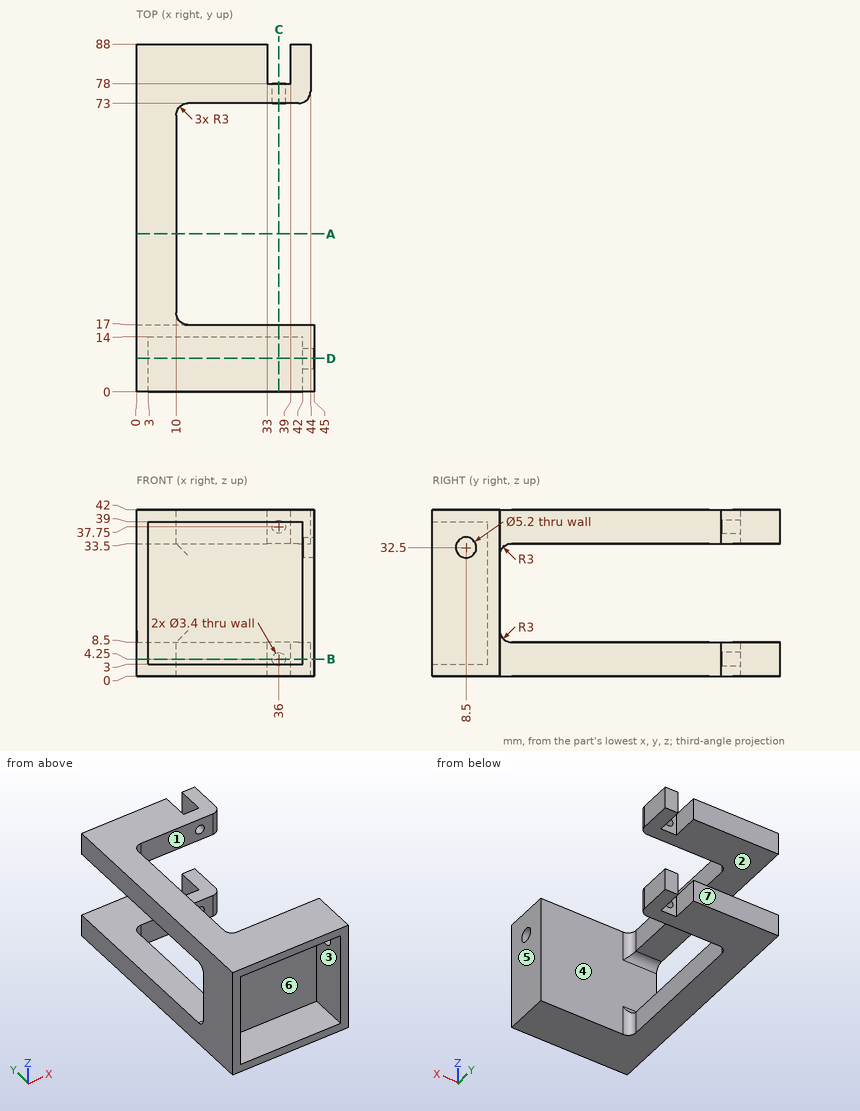
The figure shows three views and two pictorial views of one solid part (mm, origin at its lowest corner). Answer the questions. A direction names the side the tool comes from. Give positions to 0.01 mm unless a question says otherwise; leave off trailing zeros. Loops run counter-clockwise (first coordinate to the right, second up) from the corner with the lowest first, then second, coordinate; pieces in that order, holes last. Notation, with made-up numbers: (56.5, 30.25) -> (91.5, 30.25) arc R13 ccw to (91.5, 35.25) -> close; hole circle Ø7 at (43, 52). An arc over 180 degrees is marked (long way). Use a Markdown table: item, result. Add a question column.
1. Section B-B on z = 4.25 is taken. Determine the outline of the cut face in (x, y), and give its area (3 significant figures).
2. Section C-C on x = 36 is taken. Determine the outline of the cut face in (y, z).
3. Find the intervals of material crossed by probe 1 along Y at (x, z) = (32.5, 7.5); probe 2 along Y at (x, z) = (43.7, 32.5); probe 3 along Z at (x, y) = (3, 25.5), in increasing order.
4. Section D-D on y = 8.5 is taken. Determine the outline of the cut face in (x, z).
5. Determine the mould class of the marked faces 5, 6 and 7 for opening direction X: released by +X, released by -X, zero draft, split by the parting line, or undercut.
6. Flat-ended cylindrical pins translate along their axes: pin 1 Ø6 at (y, z) = (42.5, 34.5) entering from +X; pin 2 Ø3 at (x, z) = (10.5, 28) entering from -Y; pin 3 Ø1.8 at (x, z) = (37, 39.5) entering from +Y. Find the tip coordinate at first contact, or state that the pin passes through.
7. Section A-A on y = 40 is taken. Determine the outline of the cut face in (x, z), and give its area (3 significant figures).
8. For the marked faces 1, 2, 3 and 4, determine the directions among +Z, -Z, +X, -X, +Y, -Y from which every point of the face is accessible in a straight line to the end or side of a thin tool.
Results below:
| question | item | result |
|---|---|---|
| 1 | outline | (0, 0) -> (3, 0) -> (3, 14) -> (42, 14) -> (42, 0) -> (45, 0) -> (45, 17) -> (13, 17) arc R3 cw to (10, 20) -> (10, 70) arc R3 cw to (13, 73) -> (34.3, 73) -> (34.3, 78) -> (33, 78) -> (33, 88) -> (0, 88) -> close; (37.7, 73) -> (41, 73) arc R3 ccw to (44, 76) -> (44, 88) -> (39, 88) -> (39, 78) -> (37.7, 78) -> close |
| 1 | area | 1,360 mm^2 |
| 2 | outline | (0, 0) -> (17, 0) -> (17, 42) -> (0, 42) -> (0, 39) -> (14, 39) -> (14, 3) -> (0, 3) -> close; (73, 0) -> (78, 0) -> (78, 2.55) -> (73, 2.55) -> close; (73, 5.95) -> (78, 5.95) -> (78, 8.5) -> (73, 8.5) -> close; (73, 33.5) -> (78, 33.5) -> (78, 36.05) -> (73, 36.05) -> close; (73, 39.45) -> (78, 39.45) -> (78, 42) -> (73, 42) -> close |
| 3 | probe 1 | y = 14 to 17, 73 to 88 |
| 3 | probe 2 | y = 0 to 5.9, 11.1 to 17 |
| 3 | probe 3 | z = 0 to 8.5, 33.5 to 42 |
| 4 | outline | (0, 0) -> (45, 0) -> (45, 29.9) -> (42, 29.9) -> (42, 3) -> (3, 3) -> (3, 39) -> (42, 39) -> (42, 35.1) -> (45, 35.1) -> (45, 42) -> (0, 42) -> close |
| 5 | face 5 | released by +X |
| 5 | face 6 | undercut |
| 5 | face 7 | zero draft |
| 6 | pin 1 | stops at x = 10 |
| 6 | pin 2 | stops at y = 14 |
| 6 | pin 3 | stops at y = 78 |
| 7 | outline | (0, 0) -> (10, 0) -> (10, 8.5) -> (0, 8.5) -> close; (0, 33.5) -> (10, 33.5) -> (10, 42) -> (0, 42) -> close |
| 7 | area | 170 mm^2 |
| 8 | face 1 | +Z, -Z, +X |
| 8 | face 2 | +X, -X, +Y |
| 8 | face 3 | -Y |
| 8 | face 4 | +X |
